from build123d import *

# Parameters (mm, degrees)
SKETCH1_W           = 30
SKETCH1_H           = 10
BOSS_EXTRUDE1_DEPTH = 5


with BuildPart() as part:
    # Sketch1 → Boss-Extrude1 (new body)
    with BuildSketch(Plane(origin=(0, 0, 0), x_dir=(1, 0, 0), z_dir=(0, 1, 0))):
        Polygon((-22.5, -12.5), (-7.5, -12.5), (-7.5, -17.5), (7.5, -17.5), (7.5, -12.5), (22.5, -12.5), (22.5, -5.5), (27.5, -5.5), (27.5, 5.5), (22.5, 5.5), (22.5, 12.5), (7.5, 12.5), (7.5, 17.5), (-7.5, 17.5), (-7.5, 12.5), (-22.5, 12.5), (-22.5, 5.5), (-27.5, 5.5), (-27.5, -5.5), (-22.5, -5.5), align=None)
        Rectangle(SKETCH1_W, SKETCH1_H, mode=Mode.SUBTRACT)
    extrude(amount=BOSS_EXTRUDE1_DEPTH)


solid = part.part
Source: CAD feature listing. Evaluate the final solid. Frame: model axes, mm. A direction names the side the tool comes from. Give positions to 0.01 mm unless a question says otherwise; leave off trailing zeros. Write each loop counter-clockwise with the first axis right and the second up, starting at its lowest first coordinate (ties: lowest second). Pieces come first, ordered by that corner, then holes. Notation, with made-up numbers: (1.25, 15.5) -> (10.25, 15.5) arc R10 ccw to (10.25, 33.5) -> close; hole circle Ø2 at (-16.75, -29). An arc over 180 degrees is marked (long way). Write item = value, one per line.
Q1. Line query: line 1 (Z direction, x = -12.5, y = 4.6); line 2 (Z direction, x = -2.5, y = 2.6); line 3 (X direction, y = 3.75, z = 0). Output: solid intervals per line, ascending. Write a range as from..to.
Here are the results:
line_1 = -12.5..-5, 5..12.5
line_2 = -17.5..-5, 5..17.5
line_3 = -27.5..-15, 15..27.5
Q2. Reachability of faces 5 (the face through (15, 2, 12.5)), 6 (the face through (-7.5, 2, -15)), 7 (the face through (-22.5, 2, 9)), 8 (the face through (15, 2, -12.5)) from +Z, -Z, +X, -X, +Y, -Y: full face, straight path, thin tool, end or side. Return the list, or none.
Here are the results:
face_5 = +Z, +X, +Y, -Y
face_6 = -Z, -X, +Y, -Y
face_7 = +Z, -X, +Y, -Y
face_8 = -Z, +X, +Y, -Y
Q3. Mould query, pull axis X, two halves, no side actions, for faces 1 (the face through (22.5, 2, 9)), 2 (the face through (15, 2, 0)), 3 (the face through (-27.5, 2, 0)), 4 (the face through (-25, 2, -5.5)). Classes: +X half, -X half, draft (parallel to the pull), parting line (faces both ways), or undercut.
Here are the results:
face_1 = +X half
face_2 = undercut
face_3 = -X half
face_4 = draft
Q4. Cut plane A-A on z = 1. Return loops of the section in (x, y).
Here are the results:
outline = (-27.5, 0) -> (-15, 0) -> (-15, 5) -> (-27.5, 5) -> close; (15, 0) -> (27.5, 0) -> (27.5, 5) -> (15, 5) -> close
Q5. Cut plane B-B on x = -4.5. Return loops of the section in (y, z), then the cut area to 3 significant figures.
Here are the results:
outline = (0, -17.5) -> (5, -17.5) -> (5, -5) -> (0, -5) -> close; (0, 5) -> (5, 5) -> (5, 17.5) -> (0, 17.5) -> close
area = 125 mm²
Q6. Cut plane D-D on z = 9. Return loops of the section in (x, y), then the cut area to 3 significant figures.
Here are the results:
outline = (-22.5, 0) -> (22.5, 0) -> (22.5, 5) -> (-22.5, 5) -> close
area = 225 mm²
Q7. First-contact query: pin 1 (1 mm diameter, centred on y = 2, z = -11.5, fed in from -X); pin 2 (2.5 mm diameter, centred on x = -16.5, y = 2, fed in from +Z); pin 3 (1.5 mm diameter, centred on y = 2, z = -16, fed in from +X). Flat tips, straight axial feed; report the tip coordinate or a pass-through.
Here are the results:
pin_1 = -22.5
pin_2 = 12.5
pin_3 = 7.5
Q8. Cut plane C-C on y = 2.7. Return loops of the section in (x, z), then the cut area to 4 significant figures.
Here are the results:
outline = (-27.5, -5.5) -> (-22.5, -5.5) -> (-22.5, -12.5) -> (-7.5, -12.5) -> (-7.5, -17.5) -> (7.5, -17.5) -> (7.5, -12.5) -> (22.5, -12.5) -> (22.5, -5.5) -> (27.5, -5.5) -> (27.5, 5.5) -> (22.5, 5.5) -> (22.5, 12.5) -> (7.5, 12.5) -> (7.5, 17.5) -> (-7.5, 17.5) -> (-7.5, 12.5) -> (-22.5, 12.5) -> (-22.5, 5.5) -> (-27.5, 5.5) -> close; hole (-15, -5) -> (15, -5) -> (15, 5) -> (-15, 5) -> close
area = 1,085 mm²
